Geometry: final body of the model. Coordinates: model frame, mm. A direction names the side the tool comes from. Give positions to 0.01 mm unless a question says otherwise; leave off trailing zeros. Write each loop counter-clockwise with the first axis right and the second up, starting at its lowest first coordinate (ties: lowest second). Pieces come first, ordered by that corner, then holes. Notation, with made-up numbers: (62.25, 27) -> (117.25, 27) arc R20 ccw to (117.25, 57) -> close; hole circle Ø7 at (32, -9.75). An arc over 180 degrees is marked (long way). Answer in a Markdown table with one row per item. Add a question column.
Item 1: Access query for faces 1 (the flat face through (22, -2, -3)), 2 (the cylindrical face through (8.385, -0.751, -3.014)), 3 (the flat face through (10, 0, -4)). Directions: +Z, -Z, +X, -X, +Y, -Y. A direction counts if a zero-diameter tool reaches every point of the face in a straight line with its end or side. Return the directions, or none.
Item 2: Draft query along X for faces 4 (the cylindrical face through (-4, 0, -2)), 5 (the flat face through (1, 1, -2)), 6 (the flat face through (8, 0, 0)). Return one class per face: +X half, -X half, draft (parallel to the pull), parting line (faces both ways), or undercut.
Item 3: Section query D-D on y = -1.5. Output: boundary loops of the cut face in (x, z).
Item 4: Material intervals for probe 1 along Y at (x, z) = (6, -0.35); probe 2 along X at (y, z) = (1.5, -3.75); probe 3 along Y at (x, z) = (0, -2.65), sorted ascending. Write a range as from..to.
Item 5: Section query A-A on x = 6. Output: boundary loops of the cut face in (y, z).
Item 6: Section query B-B on y = -0.25. Output: boundary loops of the cut face in (x, z).
Item 7: First-contact query: P1, Ø3, axis at x = 6, y = 0, coming from the -Z side; P2, Ø2, axis at y = -2, z = -0.5, coming from the +X side; P3, Ø2, axis at y = 1.5, z = -1, coming from the +X side. Flat tips, straight axial feed; report the tip coordinate or a pass-through.
Item 8: Section query C-C on z = -1.65. Output: boundary loops of the cut face in (x, y).
```python
from build123d import *

# Parameters (mm, degrees)
F1_DEPTH = 4
F2_DEPTH = 3
F3_R     = 2.5
F4_DEPTH = 2


with BuildPart() as f1:
    # F0 (on Top) → F1 (new body)
    with BuildSketch(Plane.XY):
        with BuildLine():
            ThreePointArc((0, 1.1), (0.7778174593, 0.7778174593), (1.1, 0))
            Line((1.1, 0), (4, 0))
            ThreePointArc((4, 0), (2.8284271247, 2.8284271247), (0, 4))
            Line((0, 4), (0, 1.1))
        make_face()
        with BuildLine():
            Line((4, 0), (1.1, 0))
            ThreePointArc((1.1, 0), (-0.7778174593, -0.7778174593), (0, 1.1))
            Line((0, 1.1), (0, 4))
            ThreePointArc((0, 4), (-4, 0), (0, -4))
            ThreePointArc((0, -4), (2.8284271247, -2.8284271247), (4, 0))
        make_face()
        with BuildLine():
            ThreePointArc((0, 4), (2.8284271247, 2.8284271247), (4, 0))
            Line((4, 0), (4.9, 0))
            ThreePointArc((4.9, 0), (6, 1.1), (7.1, 0))
            Line((7.1, 0), (16, 0))
            ThreePointArc((16, 0), (17.1715728753, 2.8284271247), (20, 4))
            Line((20, 4), (0, 4))
        make_face()
        with BuildLine():
            Line((4.9, 0), (4, 0))
            ThreePointArc((4, 0), (2.8284271247, -2.8284271247), (0, -4))
            Line((0, -4), (20, -4))
            ThreePointArc((20, -4), (17.1715728753, -2.8284271247), (16, 0))
            Line((16, 0), (7.1, 0))
            ThreePointArc((7.1, 0), (6, -1.1), (4.9, 0))
        make_face()
        with BuildLine():
            Line((20, 2.1), (20, 4))
            ThreePointArc((20, 4), (17.1715728753, 2.8284271247), (16, 0))
            Line((16, 0), (17.9, 0))
            ThreePointArc((17.9, 0), (18.5150757595, 1.4849242405), (20, 2.1))
        make_face()
        with BuildLine():
            ThreePointArc((24, 0), (22.8284271247, 2.8284271247), (20, 4))
            Line((20, 4), (20, 2.1))
            ThreePointArc((20, 2.1), (21.4849242405, 1.4849242405), (22.1, 0))
            ThreePointArc((22.1, 0), (21.4849242405, -1.4849242405), (20, -2.1))
            Line((20, -2.1), (20, -4))
            ThreePointArc((20, -4), (22.8284271247, -2.8284271247), (24, 0))
        make_face()
        with BuildLine():
            ThreePointArc((16, 0), (17.1715728753, -2.8284271247), (20, -4))
            Line((20, -4), (20, -2.1))
            ThreePointArc((20, -2.1), (18.5150757595, -1.4849242405), (17.9, 0))
            Line((17.9, 0), (16, 0))
        make_face()
    extrude(amount=-F1_DEPTH)

    # F0 (on Top) → F2 (cut)
    with BuildSketch(Plane.XY):
        with BuildLine():
            ThreePointArc((16, 0), (17.1715728753, -2.8284271247), (20, -4))
            Line((20, -4), (20, -2.1))
            ThreePointArc((20, -2.1), (18.5150757595, -1.4849242405), (17.9, 0))
            Line((17.9, 0), (16, 0))
        make_face()
        with BuildLine():
            Line((20, 2.1), (20, 4))
            ThreePointArc((20, 4), (17.1715728753, 2.8284271247), (16, 0))
            Line((16, 0), (17.9, 0))
            ThreePointArc((17.9, 0), (18.5150757595, 1.4849242405), (20, 2.1))
        make_face()
        with BuildLine():
            ThreePointArc((24, 0), (22.8284271247, 2.8284271247), (20, 4))
            Line((20, 4), (20, 2.1))
            ThreePointArc((20, 2.1), (21.4849242405, 1.4849242405), (22.1, 0))
            ThreePointArc((22.1, 0), (21.4849242405, -1.4849242405), (20, -2.1))
            Line((20, -2.1), (20, -4))
            ThreePointArc((20, -4), (22.8284271247, -2.8284271247), (24, 0))
        make_face()
    extrude(amount=-F2_DEPTH, mode=Mode.SUBTRACT)

    # F3 (on face) → F4 (cut)
    with BuildSketch(Plane(origin=(0, 0, -4), x_dir=(1, 0, 0), z_dir=(0, 0, -1))):
        with Locations((6, 0)):
            Circle(F3_R)
        Circle(F3_R)
    extrude(amount=-F4_DEPTH, mode=Mode.SUBTRACT)


solid = f1.part
```
Findings below:
| question | item | result |
|---|---|---|
| 1 | face 1 | +Z, +X |
| 1 | face 2 | -Z |
| 1 | face 3 | -Z, +X, -X, +Y, -Y |
| 2 | face 4 | -X half |
| 2 | face 5 | undercut |
| 2 | face 6 | draft |
| 3 | outline | (-3.71, -4) -> (-2, -4) -> (-2, -2) -> (2, -2) -> (2, -4) -> (4, -4) -> (4, -2) -> (8, -2) -> (8, -4) -> (18.53, -4) -> (18.53, -3) -> (16.29, -3) -> (16.29, 0) -> (-3.71, 0) -> close; (21.47, -4) -> (23.71, -4) -> (23.71, -3) -> (21.47, -3) -> close |
| 4 | probe 1 | y = -4..-1.1, 1.1..4 |
| 4 | probe 2 | x = -3.71..-2, 2..4, 8..18.53, 21.47..23.71 |
| 4 | probe 3 | y = -4..-2.5, 2.5..4 |
| 5 | outline | (-4, -4) -> (-2.5, -4) -> (-2.5, -2) -> (-1.1, -2) -> (-1.1, 0) -> (-4, 0) -> close; (1.1, -2) -> (2.5, -2) -> (2.5, -4) -> (4, -4) -> (4, 0) -> (1.1, 0) -> close |
| 6 | outline | (-3.99, -4) -> (-2.49, -4) -> (-2.49, -2) -> (-1.07, -2) -> (-1.07, 0) -> (-3.99, 0) -> close; (1.07, -2) -> (2.49, -2) -> (2.49, -4) -> (3.51, -4) -> (3.51, -2) -> (4.93, -2) -> (4.93, 0) -> (1.07, 0) -> close; (7.07, -2) -> (8.49, -2) -> (8.49, -4) -> (17.91, -4) -> (17.91, -3) -> (16.01, -3) -> (16.01, 0) -> (7.07, 0) -> close; (22.09, -4) -> (23.99, -4) -> (23.99, -3) -> (22.09, -3) -> close |
| 7 | P1 | stops at z = -2 |
| 7 | P2 | stops at x = 17.35 |
| 7 | P3 | stops at x = 16.88 |
| 8 | outline | (0, -4) -> (20, -4) arc R4 cw to (20, 4) -> (0, 4) arc R4 ccw to start; hole circle Ø2.2 at (0, 0); hole circle Ø2.2 at (6, 0) |
